For this review, take the finished solid that the model builds, in its own axes (mm). A direction names the side the tool comes from. Give positions to 0.01 mm unless a question says otherwise; leave off trailing zeros. Write each loop counter-clockwise with the first axis right and the second up, starting at its lowest first coordinate (ties: lowest second). Pieces come first, ordered by that corner, then holes. Notation, with made-up numbers: M 13,-31.75 L 17,-31.75 A6 cw 17,-26.75 Z; hole C 88,13.5 d11. An arc over 180 degrees is marked long. One line per item, written item: value. Start each with the question number.
Item 1: Consider section B-B, the plane x = 5.5. Write out the cut boundary in (y, z).
Item 2: To check wall thickness, follow probe 1 along Y at (x, z) = (57.99, 4.7); probe 2 along Y at (x, z) = (39.15, 4) (3 decimals); probe 3 along X at (y, z) = (28, 4.5). State the ranges of each line that lie inside material, in increasing order.
Item 3: Tool access review of faces 3 (the face through (9, 53, 1)), 4 (the face through (85.44, 8.76, 3.97)), 5 (the face through (44, 29, 0)): name each direction out of +Z, -Z, +X, -X, +Y, -Y from which nothing blocks a thin tool from reaching the whole face with its end or side.
Item 4: Consider section A-A, the plane y = 33. Write out the cut boundary in (x, z), and give its area (3 significant figures).
Item 5: Consider section D-D, the plane y = 49. Write out the cut boundary in (x, z), and give its area (3 significant figures).
Item 6: Clearance check with flat-ended pins moving along their axes: pin 1 Ø1.2 at (x, z) = (87.5, 8.5) entering from +Y; pin 2 Ø5.5 at (x, y) = (39, 45.5) entering from +Z; pin 3 Ø4 at (x, y) = (85.5, 55) entering from -Z; pin 4 Ø1.6 at (y, z) = (53.5, 1) entering from -X. State where each tip first meets the part, or that it passes through.
Item 7: Mouldability with a two-part tool opening along Y and no side actions: class faces 1 (the face through (45, 51, 19)), 2 (the face through (86, 28, 6)) as released by +Y, released by -Y, zero draft, split by the parting line, or undercut.
Item 8: Consider section C-C, the plane x = 58. Write out the cut boundary in (y, z), and give its area (3 significant figures).
```python
from build123d import *

# Parameters (mm, degrees)
EXTRUDE045_DEPTH     = 2
SKETCH030_R          = 1.5
EXTRUDE031_DEPTH     = 4
SKETCH031_R          = 2.5
EXTRUDE030_DEPTH     = 4
SKETCH024_R          = 2.5
EXTRUDE024_DEPTH     = 2
SKETCH025_R          = 1.5
EXTRUDE027_DEPTH     = 4
SKETCH026_R          = 2.5
EXTRUDE026_DEPTH     = 4
SKETCH029_R          = 1.5
EXTRUDE029_DEPTH     = 20
EXTRUDE001_DEPTH     = 3
SKETCH_W             = 12.96
SKETCH_H             = 14.18
SKETCH_R             = 0.25
SKETCH_R_2           = 1.65
EXTRUDE_DEPTH        = 2
SKETCH013_W          = 8.5
SKETCH013_H          = 3.76
EXTRUDE013_DEPTH     = 3.54
SKETCH014_W          = 5
SKETCH014_H          = 1.5
EXTRUDE014_DEPTH     = 2.97
SKETCH012_W          = 16.69
SKETCH012_H          = 12.65
EXTRUDE012_DEPTH     = 1.66
LINK_PLACEMENT_ANGLE = 90
SKETCH027_W          = 94
SKETCH027_H          = 54
EXTRUDE025_DEPTH     = 19


with BuildPart() as extrude_controllercable_hole:
    # Sketch044 → Extrude045 (new body)
    with BuildSketch(Plane.XZ):
        with BuildLine():
            Line((-3.5, 7), (3.5, 7))
            Line((3.5, 7), (3.5, 0))
            ThreePointArc((-3.5, 0), (0, -3.5), (3.5, 0))
            Line((-3.5, 0), (-3.5, 7))
        make_face()
    extrude(amount=EXTRUDE045_DEPTH)


with BuildPart() as extrude_controllercable_hole_1:
    # Extrude045 placement: moved
    add(extrude_controllercable_hole.part.moved(Location((24, 52, 23))))


with BuildPart() as obj1:
    # Sketch030 → Extrude031 (new body)
    with BuildSketch(Plane.XY):
        with Locations((2.15, 7.435)):
            Circle(SKETCH030_R)
        with Locations((10.81, 7.435)):
            Circle(SKETCH030_R)
    extrude(amount=EXTRUDE031_DEPTH)


with BuildPart() as obj2:
    # Sketch031 → Extrude030 (new body)
    with BuildSketch(Plane.XY):
        with Locations((2.15, 7.435)):
            Circle(SKETCH031_R)
        with Locations((10.81, 7.435)):
            Circle(SKETCH031_R)
    extrude(amount=EXTRUDE030_DEPTH)

    # Cut004: cut obj1
    add(obj1.part, mode=Mode.SUBTRACT)


with BuildPart() as obj2_1:
    # Cut004 placement: moved
    add(obj2.part.moved(Location((37, 37.9, 2))))


with BuildPart() as extrude_controllercase_base:
    # Sketch024 → Extrude024 (new body)
    with BuildSketch(Plane.XY):
        with BuildLine():
            Line((0, 0), (90, 0))
            Line((90, 0), (90, 50))
            Line((90, 50), (90, 55))
            ThreePointArc((90, 55), (85.5, 59.5), (81, 55))
            Line((81, 50), (81, 55))
            Line((81, 50), (9, 50))
            Line((9, 50), (9, 55))
            ThreePointArc((9, 55), (4.5, 59.5), (0, 55))
            Line((0, 50), (0, 55))
            Line((0, 50), (0, 0))
        make_face()
        with Locations((85.5, 55)):
            Circle(SKETCH024_R, mode=Mode.SUBTRACT)
        with Locations((4.5, 55)):
            Circle(SKETCH024_R, mode=Mode.SUBTRACT)
    extrude(amount=EXTRUDE024_DEPTH)


with BuildPart() as extrude_mainboardcase_joystick_hole:
    # Sketch025 → Extrude027 (new body)
    with BuildSketch(Plane(origin=(53, 3, 0), x_dir=(1, 0, 0), z_dir=(0, 0, 1))):
        with Locations((-48, 19.88)):
            Circle(SKETCH025_R)
        with Locations((-21.99, 19.88)):
            Circle(SKETCH025_R)
        with Locations((-48.01, 0.31)):
            Circle(SKETCH025_R)
        with Locations((-21.99, 0.31)):
            Circle(SKETCH025_R)
    extrude(amount=EXTRUDE027_DEPTH)


with BuildPart() as fusion_controllercase_base:
    # Sketch026 → Extrude026 (new body)
    with BuildSketch(Plane.XY):
        with Locations((5, 22.88)):
            Circle(SKETCH026_R)
        with Locations((31.01, 22.88)):
            Circle(SKETCH026_R)
        with Locations((31.01, 3.31)):
            Circle(SKETCH026_R)
        with Locations((4.99, 3.31)):
            Circle(SKETCH026_R)
    extrude(amount=EXTRUDE026_DEPTH)

    # Cut001: cut Extrude_MainBoardCase_JoyStick_Hole
    add(extrude_mainboardcase_joystick_hole.part, mode=Mode.SUBTRACT)


with BuildPart() as fusion_controllercase_base_1:
    # Cut001 placement: moved
    add(fusion_controllercase_base.part.moved(Location((53, 5, 2))))

    # Fusion007: union obj2, Extrude_ControllerCase_Base
    add(obj2_1.part)
    add(extrude_controllercase_base.part)


with BuildPart() as obj3:
    # Sketch029 → Extrude029 (new body)
    with BuildSketch(Plane.XY):
        with Locations((1, 49)):
            Circle(SKETCH029_R)
        with Locations((1, 1)):
            Circle(SKETCH029_R)
        with Locations((89, 1)):
            Circle(SKETCH029_R)
        with Locations((89, 49)):
            Circle(SKETCH029_R)
    extrude(amount=EXTRUDE029_DEPTH)


with BuildPart() as obj3_1:
    # Extrude029 placement: moved
    add(obj3.part.moved(Location((0, 0, 2))))


with BuildPart() as obj4:
    # Sketch001 → Extrude001 (new body)
    with BuildSketch(Plane.XY):
        Polygon((10.18, 14.18), (10.18, 8.98), (2.78, 8.98), (2.78, 14.18), (6.48, 14.18), align=None)
    extrude(amount=EXTRUDE001_DEPTH)


with BuildPart() as obj4_1:
    # Extrude001 placement: moved
    add(obj4.part.moved(Location((0, 0, 2))))


with BuildPart() as obj5:
    # Sketch → Extrude (new body)
    with BuildSketch(Plane.XY):
        with Locations((6.48, 7.09)):
            Rectangle(SKETCH_W, SKETCH_H)
        with Locations((1, 1)):
            Circle(SKETCH_R, mode=Mode.SUBTRACT)
        with Locations((3.74, 1)):
            Circle(SKETCH_R, mode=Mode.SUBTRACT)
        with Locations((6.48, 1)):
            Circle(SKETCH_R, mode=Mode.SUBTRACT)
        with Locations((9.22, 1)):
            Circle(SKETCH_R, mode=Mode.SUBTRACT)
        with Locations((11.96, 1)):
            Circle(SKETCH_R, mode=Mode.SUBTRACT)
        with Locations((2.15, 7.435)):
            Circle(SKETCH_R_2, mode=Mode.SUBTRACT)
        with Locations((10.81, 7.435)):
            Circle(SKETCH_R_2, mode=Mode.SUBTRACT)
    extrude(amount=EXTRUDE_DEPTH)

    # Fusion: union obj4
    add(obj4_1.part)


with BuildPart() as obj5_1:
    # Fusion placement: moved
    add(obj5.part.moved(Location((-20, 0, 0))))


with BuildPart() as obj5_2:
    # Link002 placement: moved
    add(obj5_1.part.moved(Location((57, 37.9, 6))))


with BuildPart() as extrude_switch_house:
    # Sketch013 → Extrude013 (new body)
    with BuildSketch(Plane.XY):
        with Locations((4.25, 1.88)):
            Rectangle(SKETCH013_W, SKETCH013_H)
    extrude(amount=EXTRUDE013_DEPTH)


with BuildPart() as extrude_switch:
    # Sketch014 → Extrude014 (new body)
    with BuildSketch(Plane.XY):
        with Locations((4.25, 1.88)):
            Rectangle(SKETCH014_W, SKETCH014_H)
    extrude(amount=EXTRUDE014_DEPTH)


with BuildPart() as extrude_switch_1:
    # Extrude014 placement: moved
    add(extrude_switch.part.moved(Location((0, 0, 3.54))))


with BuildPart() as obj6:
    # Sketch012 → Extrude012 (new body)
    with BuildSketch(Plane(origin=(4, 2, 0), x_dir=(1, 0, 0), z_dir=(0, 0, 1))):
        Rectangle(SKETCH012_W, SKETCH012_H)
    extrude(amount=-EXTRUDE012_DEPTH)

    # Fusion004: union Extrude_Switch_house, Extrude_Switch_
    add(extrude_switch_house.part)
    add(extrude_switch_1.part)


with BuildPart() as obj6_1:
    # Fusion004 placement: moved
    add(obj6.part.moved(Location((-150, 0, 0))))


with BuildPart() as obj6_2:
    # Link placement: moved
    add(obj6_1.part.moved(Location((89, 37, -136))).rotate(Axis((89, 37, -136), (0, 1, 0)), LINK_PLACEMENT_ANGLE))


with BuildPart() as cut_controllercase_bottom:
    # Sketch027 → Extrude025 (new body)
    with BuildSketch(Plane.XY):
        with Locations((45, 25)):
            Rectangle(SKETCH027_W, SKETCH027_H)
        Polygon((86, 50), (4, 50), (4, 46), (0, 46), (0, 4), (4, 4), (4, 0), (86, 0), (86, 4), (90, 4), (90, 46), (86, 46), align=None, mode=Mode.SUBTRACT)
    extrude(amount=EXTRUDE025_DEPTH)

    # Cut005: cut obj6
    add(obj6_2.part, mode=Mode.SUBTRACT)

    # Cut006: cut obj5
    add(obj5_2.part, mode=Mode.SUBTRACT)

    # Cut007: cut obj3
    add(obj3_1.part, mode=Mode.SUBTRACT)

    # Fusion008: union Fusion_ControllerCase_Base
    add(fusion_controllercase_base_1.part)

    # Cut011: cut Extrude_ControllerCable_Hole
    add(extrude_controllercable_hole_1.part, mode=Mode.SUBTRACT)


solid = cut_controllercase_bottom.part
```
Model answer:
1. outline: M -2,0 L 52.71,0 L 52.71,2 L 52,2 L 52,19 L 50,19 L 50,2 L 0,2 L 0,19 L -2,19 Z; M 57.29,0 L 59.39,0 L 59.39,2 L 57.29,2 Z
2. probe 1: y = -2 to 0, 5.81 to 6.81, 9.81 to 10.81, 25.38 to 26.38, 29.38 to 30.38, 50 to 52
2. probe 2: y = -2 to 0, 42.835 to 43.835, 46.835 to 47.835, 50 to 52
2. probe 3: x = -2 to 0, 55.5 to 56.5, 59.5 to 60.5, 81.51 to 82.51, 85.51 to 86.51, 90 to 92
3. face 3: +Z, -Z, +Y
3. face 4: +Z
3. face 5: -Z, +X, -X, +Y, -Y
4. outline: M -2,0 L 92,0 L 92,19 L 90,19 L 90,2 L 0,2 L 0,19 L -2,19 Z
4. area: 256 mm2
5. outline: M -2,0 L 92,0 L 92,19 L 90.5,19 L 90.5,2 L 87.5,2 L 87.5,19 L 86,19 L 86,2 L 4,2 L 4,19 L 2.5,19 L 2.5,2 L -0.5,2 L -0.5,19 L -2,19 Z
5. area: 290 mm2
6. pin 1: stops at y = 52
6. pin 2: stops at z = 6
6. pin 3: passes through
6. pin 4: stops at x = 0
7. face 1: zero draft
7. face 2: undercut
8. outline: M -2,0 L 52,0 L 52,19 L 50,19 L 50,2 L 30.38,2 L 30.38,6 L 29.38,6 L 29.38,2 L 26.38,2 L 26.38,6 L 25.38,6 L 25.38,2 L 10.81,2 L 10.81,6 L 9.81,6 L 9.81,2 L 6.81,2 L 6.81,6 L 5.81,6 L 5.81,2 L 0,2 L 0,19 L -2,19 Z
8. area: 192 mm2
